from build123d import *

# Parameters (mm, degrees)
F1_DEPTH = 40
F0_R     = 2
F2_DEPTH = 1
F3_DEPTH = 2
F4_DEPTH = 1


with BuildPart() as f1:
    # F0 (on Top) → F1 (new body)
    with BuildSketch(Plane.XY):
        with BuildLine():
            Line((23.4693709612, 14.670217514), (-112.5306290388, 14.670217514))
            ThreePointArc((-112.5306290388, 14.670217514), (-116.0661629447, 13.20575142), (-117.5306290388, 9.670217514))
            Line((-117.5306290388, 9.670217514), (-117.5306290388, -36.329782486))
            ThreePointArc((-117.5306290388, -36.329782486), (-116.0661629447, -39.8653163919), (-112.5306290388, -41.329782486))
            Line((-112.5306290388, -41.329782486), (23.4693709612, -41.329782486))
            ThreePointArc((23.4693709612, -41.329782486), (27.0049048671, -39.8653163919), (28.4693709612, -36.329782486))
            Line((28.4693709612, -36.329782486), (28.4693709612, 9.670217514))
            ThreePointArc((28.4693709612, 9.670217514), (27.0049048671, 13.20575142), (23.4693709612, 14.670217514))
        make_face()
        with BuildLine():
            ThreePointArc((-114.5306290388, 9.670217514), (-113.9448426012, 11.0844310764), (-112.5306290388, 11.670217514))
            Line((-112.5306290388, 11.670217514), (23.4693709612, 11.670217514))
            ThreePointArc((23.4693709612, 11.670217514), (24.8835845236, 11.0844310764), (25.4693709612, 9.670217514))
            Line((25.4693709612, 9.670217514), (25.4693709612, -36.329782486))
            ThreePointArc((25.4693709612, -36.329782486), (24.8835845236, -37.7439960483), (23.4693709612, -38.329782486))
            Line((23.4693709612, -38.329782486), (-112.5306290388, -38.329782486))
            ThreePointArc((-112.5306290388, -38.329782486), (-113.9448426012, -37.7439960483), (-114.5306290388, -36.329782486))
            Line((-114.5306290388, -36.329782486), (-114.5306290388, 9.670217514))
        make_face(mode=Mode.SUBTRACT)
    extrude(amount=-F1_DEPTH)



with BuildPart() as f2:
    # F0 (on Top) → F2 (new body)
    with BuildSketch(Plane.XY):
        with BuildLine():
            ThreePointArc((-124.5306290388, 31.670217514), (-131.6016968507, 28.7412853259), (-134.5306290388, 21.670217514))
            Line((-134.5306290388, 21.670217514), (-134.5306290388, -48.329782486))
            ThreePointArc((-134.5306290388, -48.329782486), (-131.6016968507, -55.4008502978), (-124.5306290388, -58.329782486))
            Line((-124.5306290388, -58.329782486), (35.4693709612, -58.329782486))
            ThreePointArc((35.4693709612, -58.329782486), (42.5404387731, -55.4008502978), (45.4693709612, -48.329782486))
            Line((45.4693709612, -48.329782486), (45.4693709612, 21.670217514))
            ThreePointArc((45.4693709612, 21.670217514), (42.5404387731, 28.7412853259), (35.4693709612, 31.670217514))
            Line((35.4693709612, 31.670217514), (-124.5306290388, 31.670217514))
        make_face()
        with Locations((-123.5306290388, -47.329782486)):
            Circle(F0_R, mode=Mode.SUBTRACT)
        with Locations((35.4693709612, -48.329782486)):
            Circle(F0_R, mode=Mode.SUBTRACT)
        with Locations((-124.5306290388, 21.670217514)):
            Circle(F0_R, mode=Mode.SUBTRACT)
        with BuildLine():
            ThreePointArc((-117.5306290388, 9.670217514), (-116.0661629447, 13.20575142), (-112.5306290388, 14.670217514))
            Line((-112.5306290388, 14.670217514), (23.4693709612, 14.670217514))
            ThreePointArc((23.4693709612, 14.670217514), (27.0049048671, 13.20575142), (28.4693709612, 9.670217514))
            Line((28.4693709612, 9.670217514), (28.4693709612, -36.329782486))
            ThreePointArc((28.4693709612, -36.329782486), (27.0049048671, -39.8653163919), (23.4693709612, -41.329782486))
            Line((23.4693709612, -41.329782486), (-112.5306290388, -41.329782486))
            ThreePointArc((-112.5306290388, -41.329782486), (-116.0661629447, -39.8653163919), (-117.5306290388, -36.329782486))
            Line((-117.5306290388, -36.329782486), (-117.5306290388, 9.670217514))
        make_face(mode=Mode.SUBTRACT)
        with Locations((35.4693709612, 21.670217514)):
            Circle(F0_R, mode=Mode.SUBTRACT)
    extrude(amount=F2_DEPTH)


with BuildPart() as f1_1:
    add(f1.part)

    add(f2.part)  # F3 merges F2
    # F0 (on Top) → F3 (join)
    with BuildSketch(Plane.XY):
        with BuildLine():
            ThreePointArc((-124.5306290388, 31.670217514), (-131.6016968507, 28.7412853259), (-134.5306290388, 21.670217514))
            Line((-134.5306290388, 21.670217514), (-134.5306290388, -48.329782486))
            ThreePointArc((-134.5306290388, -48.329782486), (-131.6016968507, -55.4008502978), (-124.5306290388, -58.329782486))
            Line((-124.5306290388, -58.329782486), (35.4693709612, -58.329782486))
            ThreePointArc((35.4693709612, -58.329782486), (42.5404387731, -55.4008502978), (45.4693709612, -48.329782486))
            Line((45.4693709612, -48.329782486), (45.4693709612, 21.670217514))
            ThreePointArc((45.4693709612, 21.670217514), (42.5404387731, 28.7412853259), (35.4693709612, 31.670217514))
            Line((35.4693709612, 31.670217514), (-124.5306290388, 31.670217514))
        make_face()
        with Locations((-123.5306290388, -47.329782486)):
            Circle(F0_R, mode=Mode.SUBTRACT)
        with Locations((35.4693709612, -48.329782486)):
            Circle(F0_R, mode=Mode.SUBTRACT)
        with Locations((-124.5306290388, 21.670217514)):
            Circle(F0_R, mode=Mode.SUBTRACT)
        with BuildLine():
            ThreePointArc((-117.5306290388, 9.670217514), (-116.0661629447, 13.20575142), (-112.5306290388, 14.670217514))
            Line((-112.5306290388, 14.670217514), (23.4693709612, 14.670217514))
            ThreePointArc((23.4693709612, 14.670217514), (27.0049048671, 13.20575142), (28.4693709612, 9.670217514))
            Line((28.4693709612, 9.670217514), (28.4693709612, -36.329782486))
            ThreePointArc((28.4693709612, -36.329782486), (27.0049048671, -39.8653163919), (23.4693709612, -41.329782486))
            Line((23.4693709612, -41.329782486), (-112.5306290388, -41.329782486))
            ThreePointArc((-112.5306290388, -41.329782486), (-116.0661629447, -39.8653163919), (-117.5306290388, -36.329782486))
            Line((-117.5306290388, -36.329782486), (-117.5306290388, 9.670217514))
        make_face(mode=Mode.SUBTRACT)
        with Locations((35.4693709612, 21.670217514)):
            Circle(F0_R, mode=Mode.SUBTRACT)
    extrude(amount=-F3_DEPTH)

    # F0 (on Top) → F4 (join)
    with BuildSketch(Plane.XY):
        with BuildLine():
            Line((23.4693709612, 14.670217514), (-112.5306290388, 14.670217514))
            ThreePointArc((-112.5306290388, 14.670217514), (-116.0661629447, 13.20575142), (-117.5306290388, 9.670217514))
            Line((-117.5306290388, 9.670217514), (-117.5306290388, -36.329782486))
            ThreePointArc((-117.5306290388, -36.329782486), (-116.0661629447, -39.8653163919), (-112.5306290388, -41.329782486))
            Line((-112.5306290388, -41.329782486), (23.4693709612, -41.329782486))
            ThreePointArc((23.4693709612, -41.329782486), (27.0049048671, -39.8653163919), (28.4693709612, -36.329782486))
            Line((28.4693709612, -36.329782486), (28.4693709612, 9.670217514))
            ThreePointArc((28.4693709612, 9.670217514), (27.0049048671, 13.20575142), (23.4693709612, 14.670217514))
        make_face()
        with BuildLine():
            ThreePointArc((-114.5306290388, 9.670217514), (-113.9448426012, 11.0844310764), (-112.5306290388, 11.670217514))
            Line((-112.5306290388, 11.670217514), (23.4693709612, 11.670217514))
            ThreePointArc((23.4693709612, 11.670217514), (24.8835845236, 11.0844310764), (25.4693709612, 9.670217514))
            Line((25.4693709612, 9.670217514), (25.4693709612, -36.329782486))
            ThreePointArc((25.4693709612, -36.329782486), (24.8835845236, -37.7439960483), (23.4693709612, -38.329782486))
            Line((23.4693709612, -38.329782486), (-112.5306290388, -38.329782486))
            ThreePointArc((-112.5306290388, -38.329782486), (-113.9448426012, -37.7439960483), (-114.5306290388, -36.329782486))
            Line((-114.5306290388, -36.329782486), (-114.5306290388, 9.670217514))
        make_face(mode=Mode.SUBTRACT)
        with BuildLine():
            Line((23.4693709612, 11.670217514), (-112.5306290388, 11.670217514))
            ThreePointArc((-112.5306290388, 11.670217514), (-113.9448426012, 11.0844310764), (-114.5306290388, 9.670217514))
            Line((-114.5306290388, 9.670217514), (-114.5306290388, -36.329782486))
            ThreePointArc((-114.5306290388, -36.329782486), (-113.9448426012, -37.7439960483), (-112.5306290388, -38.329782486))
            Line((-112.5306290388, -38.329782486), (23.4693709612, -38.329782486))
            ThreePointArc((23.4693709612, -38.329782486), (24.8835845236, -37.7439960483), (25.4693709612, -36.329782486))
            Line((25.4693709612, -36.329782486), (25.4693709612, 9.670217514))
            ThreePointArc((25.4693709612, 9.670217514), (24.8835845236, 11.0844310764), (23.4693709612, 11.670217514))
        make_face()
    extrude(amount=F4_DEPTH)


solid = f1_1.part
Geometry check sheet. Reference: the model listing, model coordinates, mm. A direction names the side the tool comes from. Give positions to 0.01 mm unless a question says otherwise; leave off trailing zeros. Write each loop counter-clockwise with the first axis right and the second up, starting at its lowest first coordinate (ties: lowest second). Pieces come first, ordered by that corner, then holes.
1) Set-up check for faces 1 (the face through (-116.1, -39.83, -20.73)), 2 (the face through (-117.531, -13, -21)), 3 (the face through (25.469, -13, -20)): record each of +Z, -Z, +X, -X, +Y, -Y from which the full face is reachable in a straight line by a thin tool's end or side.
Values follow:
face 1: -Z, -X, -Y
face 2: -Z, -X, +Y, -Y
face 3: -Z
2) Release check for a two-part mould opening along Y. For faces 4 (the face through (-44, 14.67, -21)), 5 (the face through (-44, -38.33, -20)), 6 (the face through (-45, -41.33, -21)) record: released by +Y, released by -Y, zero draft, split by the parting line, or undercut.
Values follow:
face 4: released by +Y
face 5: undercut
face 6: released by -Y
3) Thickness scan on line 1 (X direction, y = -35.5, z = -0.5); line 2 (X direction, y = -21.5, z = -4); line 3 (Y direction, x = -102, z = -1.5). Record the ranges inside material, lowest first.
Values follow:
line 1: x = -134.53 to -114.53, 25.47 to 45.47
line 2: x = -117.53 to -114.53, 25.47 to 28.47
line 3: y = -58.33 to -38.33, 11.67 to 31.67
4) Go/stop test with flat-tipped pins: pin 1 Ø2 at (y, z) = (-6, -24.5) entering from -X; pin 2 Ø6.5 at (x, y) = (35.47, 21.67) entering from -Z; pin 3 Ø12 at (x, z) = (-52, -29.5) entering from +Y. Record where each tip stops, or that it passes through.
Values follow:
pin 1: stops at x = -117.53
pin 2: stops at z = -2
pin 3: stops at y = 14.67
5) Cross-section at C-C (y = -10). Record the boundary of the cut face in (x, z), plus the area to 3 significant figures.
Values follow:
outline: (-134.53, -2) - (-117.53, -2) - (-117.53, -40) - (-114.53, -40) - (-114.53, 0) - (25.47, 0) - (25.47, -40) - (28.47, -40) - (28.47, -2) - (45.47, -2) - (45.47, 1) - (-134.53, 1) - close
area: 488 mm2
6) Cross-section at D-D (x = 31.5). Record the boundary of the cut face in (y, z).
Values follow:
outline: (-58.33, -2) - (31.67, -2) - (31.67, 1) - (-58.33, 1) - close
7) Cross-section at A-A (z = -21). Record the boundary of the cut face in (x, y), plus the area to 3 significant figures.
Values follow:
outline: (-117.53, -36.33) arc R5 ccw to (-112.53, -41.33) - (23.47, -41.33) arc R5 ccw to (28.47, -36.33) - (28.47, 9.67) arc R5 ccw to (23.47, 14.67) - (-112.53, 14.67) arc R5 ccw to (-117.53, 9.67) - close; hole (-114.53, -36.33) arc R2 ccw to (-112.53, -38.33) - (23.47, -38.33) arc R2 ccw to (25.47, -36.33) - (25.47, 9.67) arc R2 ccw to (23.47, 11.67) - (-112.53, 11.67) arc R2 ccw to (-114.53, 9.67) - close
area: 1,160 mm2
8) Cross-section at B-B (x = 0.5). Record the boundary of the cut face in (y, z), plus the area to 3 significant figures.
Values follow:
outline: (-58.33, -2) - (-41.33, -2) - (-41.33, -40) - (-38.33, -40) - (-38.33, 0) - (11.67, 0) - (11.67, -40) - (14.67, -40) - (14.67, -2) - (31.67, -2) - (31.67, 1) - (-58.33, 1) - close
area: 398 mm2
